```python
from build123d import *

# Parameters (mm, degrees)
BOSS_EXTRUDE1_DEPTH = 5
SKETCH3_W           = 5
SKETCH3_H           = 15
BOSS_EXTRUDE2_DEPTH = 5
SKETCH4_R           = 4.5
CUT_EXTRUDE1_DEPTH  = 178.20653008
SKETCH5_W           = 5
SKETCH5_H           = 15
CUT_EXTRUDE2_DEPTH  = 178.20653008
CUT_EXTRUDE3_DEPTH  = 178.20653008


with BuildPart() as part:
    # Sketch1 → Boss-Extrude1 (new body)
    with BuildSketch(Plane.XY):
        with BuildLine():
            Line((0, 0), (67.568382456, 0))
            Line((67.568382456, 0), (15.5, 119.786515986))
            Line((15.5, 119.786515986), (10.5, 119.786515986))
            Line((10.5, 119.786515986), (10.5, 128.17540896))
            ThreePointArc((10.5, 128.17540896), (6.5, 132.647544915), (10.5, 137.11968087))
            Line((10.5, 137.11968087), (10.5, 162.648799484))
            Line((10.5, 162.648799484), (0, 162.648799484))
            Line((0, 162.648799484), (0, 0))
        make_face()
    boss_extrude1 = extrude(amount=BOSS_EXTRUDE1_DEPTH)

    # Sketch3 → Boss-Extrude2 (add)
    with BuildSketch(Plane.XY.offset(5)):
        Polygon((65.57516115, 4.585528195), (59.595497232, 18.34211278), (64.181025427, 20.335334085), (70.160689345, 6.578749501), align=None)
        Polygon((27.703956339, 91.710563898), (21.724292422, 105.467148482), (26.309820617, 107.460369788), (32.289484534, 93.703785203), align=None)
        with Locations((13, 148.148799484)):
            Rectangle(SKETCH3_W, SKETCH3_H)
    boss_extrude2 = extrude(amount=-BOSS_EXTRUDE2_DEPTH)

    # Mirror1: Boss-Extrude1, Boss-Extrude2 across plane
    add(boss_extrude1.mirror(Plane(origin=(0, 162.648799484, 5), x_dir=(0, 0, 1), z_dir=(1, 0, 0))))
    add(boss_extrude2.mirror(Plane(origin=(0, 162.648799484, 5), x_dir=(0, 0, 1), z_dir=(1, 0, 0))))

    # Sketch4 → Cut-Extrude1 (cut, through all)
    with BuildSketch(Plane.XY.offset(5)):
        with Locations((0, 153.648852717)):
            Circle(SKETCH4_R)
        with Locations((-59.99258678, 8.648878597)):
            Circle(SKETCH4_R)
        with Locations((59.99258678, 8.648878597)):
            Circle(SKETCH4_R)
    extrude(amount=-CUT_EXTRUDE1_DEPTH, mode=Mode.SUBTRACT)

    # Sketch5 → Cut-Extrude2 (cut, through all)
    with BuildSketch(Plane.XY.offset(5)):
        with Locations((13, 42.5)):
            Rectangle(SKETCH5_W, SKETCH5_H)
        with Locations((-13, 42.5)):
            Rectangle(SKETCH5_W, SKETCH5_H)
    extrude(amount=-CUT_EXTRUDE2_DEPTH, mode=Mode.SUBTRACT)

    # Sketch6 → Cut-Extrude3 (cut, through all)
    with BuildSketch(Plane.XY.offset(5)):
        with BuildLine():
            Line((-52.677576554, 26.731708191), (-51.481643771, 29.483025108))
            ThreePointArc((-51.481643771, 29.483025108), (-50.16589387, 30.001486486), (-49.647432493, 28.685736586))
            Line((-49.647432493, 28.685736586), (-50.843365276, 25.934419669))
            ThreePointArc((-50.843365276, 25.934419669), (-52.159115176, 25.415958291), (-52.677576554, 26.731708191))
        make_face()
        with BuildLine():
            Line((-22.560773856, 96.017264948), (-21.364841072, 98.768581865))
            ThreePointArc((-21.364841072, 98.768581865), (-20.049091172, 99.287043243), (-19.530629794, 97.971293343))
            Line((-19.530629794, 97.971293343), (-20.726562578, 95.219976426))
            ThreePointArc((-20.726562578, 95.219976426), (-22.042312478, 94.701515048), (-22.560773856, 96.017264948))
        make_face()
    cut_extrude3 = extrude(amount=-CUT_EXTRUDE3_DEPTH, mode=Mode.SUBTRACT)

    # Mirror2: Cut-Extrude3 across plane
    add(cut_extrude3.mirror(Plane(origin=(0, 0, 0), x_dir=(0, 0, 1), z_dir=(1, 0, 0))), mode=Mode.SUBTRACT)


solid = part.part
```
Can you work these out from the model? Positions are in its coordinate system, mm. A direction names the side the tool comes from. Round coordinates to 2 decimals unless told otherwise and drop trailing zeros. Order: outer loops, then holes, each group sorted by start corner. A loop starts at its lowest first (then second) coordinate and runs counter-clockwise, first axis right, second up. Notation, with made-up numbers: (62, 58) -> (120, 58) arc R36 ccw to (120, 97) -> close; hole circle Ø6 at (-14, 10). An arc over 180 degrees is marked (long way). Return JSON: item names as keys, results as strings. Group by question number.
1. Will these pins go through, and if not, where does the flat tip stop? pin 1 (1.8 mm diameter, centred on y = 138.5, z = 2, fed in from +X); pin 2 (1.5 mm diameter, centred on x = 12, z = 3, fed in from +Y).
2. If we section it at A-A, the plane x = 0: Write out the boundary of the cut face in (y, z).
3. If we section it at B-B, the plane y = 63: Write out the boundary of the cut face in (x, z).
4. I need wall thicknesses on line 1 (Y direction, x = 0, z = 1.05); line 2 (Y direction, x = 14, z = 2.55); line 3 (X direction, y = 122.5, z = 3.1). Which ranges of each line are inside material? Lowest first, please. Write a range as [from, to].
5. If we section it at D-D, the plane x = 38: Write out the boundary of the cut face in (y, z).
6. We'd pull the mould along Y, two halves only. Please class faces 6 (the face through (10.5, 139, 2)), 7 (the face through (-61.856, 19.325, 2.535)), 8 (the face through (1, 0, 2)): released by +Y, released by -Y, zero draft, split by the parting line, or undercut.
7. Which directions (+Z, -Z, +X, -X, +Y, -Y) give clear straight access to the entire face, cutting with the end or side of a thin tool? Please do faces 1 (the face through (13, 50, 3)), 2 (the face through (-30.03, 92.72, 2.54)), 3 (the face through (-10.5, 159, 2)), 4 (the face through (10.5, 159, 2)), 5 (the face through (30.03, 92.72, 2.54)).
8. If we section it at C-C, the plane z = 3.2: Count the separate pieces of the cut face and the enclosed holes in it, then the cut area to 3 significant figures.
Output values:
{
 "1": {"pin 1": "x = 10.5", "pin 2": "y = 155.65"},
 "2": {"outline": "(0, 0) -> (149.15, 0) -> (149.15, 5) -> (0, 5) -> close; (158.15, 0) -> (162.65, 0) -> (162.65, 5) -> (158.15, 5) -> close"},
 "3": {"outline": "(-40.18, 0) -> (40.18, 0) -> (40.18, 5) -> (-40.18, 5) -> close"},
 "4": {"line 1": "[0, 149.15], [158.15, 162.65]", "line 2": "[0, 35], [50, 119.79], [140.65, 155.65]", "line 3": "[-10.5, 10.5]"},
 "5": {"outline": "(0, 0) -> (68.02, 0) -> (68.02, 5) -> (0, 5) -> close"},
 "6": {"face 6": "undercut", "face 7": "released by +Y", "face 8": "released by -Y"},
 "7": {"face 1": "+Z, -Z", "face 2": "+Z, -Z, -X", "face 3": "+Z, -Z, -X, +Y", "face 4": "+Z, -Z, +X, +Y", "face 5": "+Z, -Z, +X"},
 "8": {"separate pieces": "1", "enclosed holes": "9", "area": "10,900 mm²"}
}
